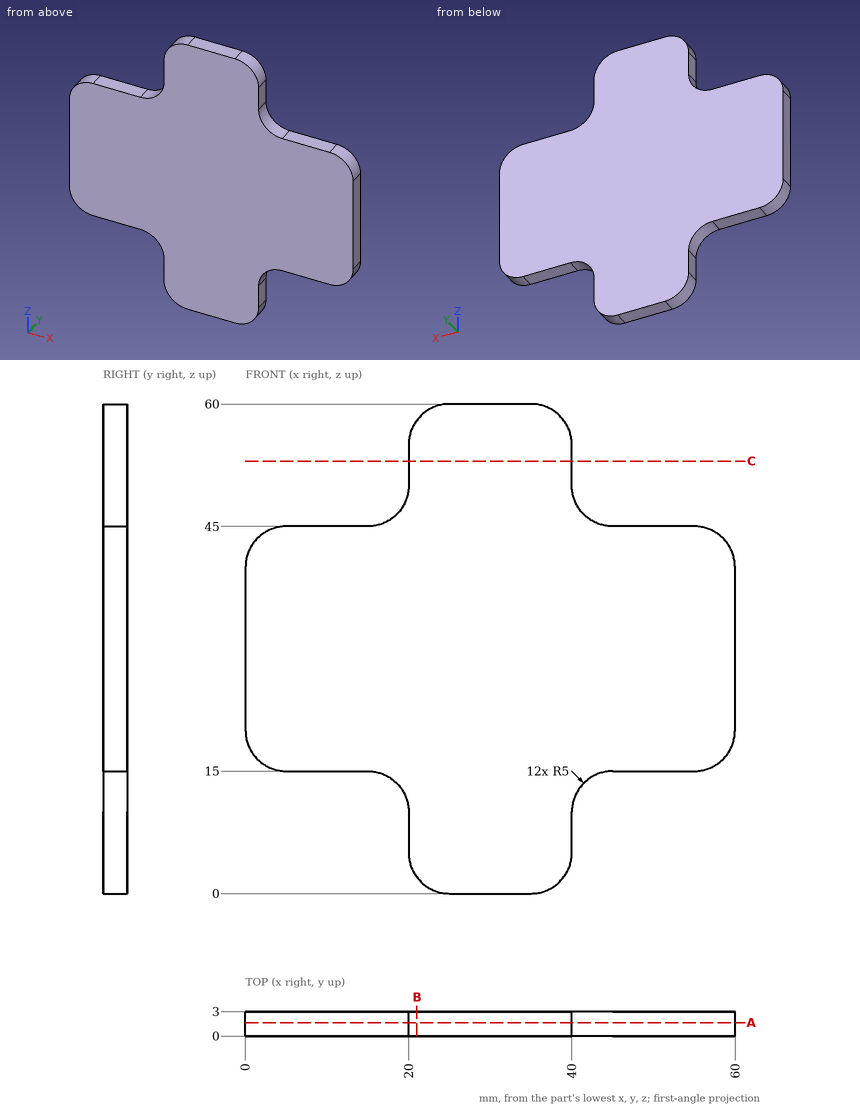
Geometry: see drawing. Coordinates: mm, zero at the bounding-box minimum. Give positions to 0.01 mm unless a question says otherwise; leave off trailing zeros. Order: outer loops, then holes, each group sorted by start corner. A loop starts at its lowest first (then second) coordinate and runs counter-clockwise, first axis right, second up. Notation, with made-up numbers: (3.25, 43) -> (37.25, 43) arc R13 cw to (37.25, 59) -> close; hole circle Ø10 at (38.5, 15.25). An arc over 180 degrees is marked (long way). Write each question's results on one line, items separated by ' | '.
1) Cut plane B-B (x = 21). Output: boundary loops of the cut face in (y, z), and give its area (3 significant figures).
Geometry says:
outline: (0, 2) -> (3, 2) -> (3, 58) -> (0, 58) -> close | area: 168 mm²
2) First-contact query: pin 1 Ø6 at (x, z) = (22, 53) entering from -Y; pin 2 Ø1.5 at (x, y) = (8.5, 1) entering from +Z. Flat tips, straight axial feed; report the tip coordinate or a pass-through.
Geometry says:
pin 1: stops at y = 0 | pin 2: stops at z = 45
3) Cut plane A-A (y = 1.65). Output: boundary loops of the cut face in (x, z), and give its area (3 significant figures).
Geometry says:
outline: (0, 20) arc R5 ccw to (5, 15) -> (15, 15) arc R5 cw to (20, 10) -> (20, 5) arc R5 ccw to (25, 0) -> (35, 0) arc R5 ccw to (40, 5) -> (40, 10) arc R5 cw to (45, 15) -> (55, 15) arc R5 ccw to (60, 20) -> (60, 40) arc R5 ccw to (55, 45) -> (45, 45) arc R5 cw to (40, 50) -> (40, 55) arc R5 ccw to (35, 60) -> (25, 60) arc R5 ccw to (20, 55) -> (20, 50) arc R5 cw to (15, 45) -> (5, 45) arc R5 ccw to (0, 40) -> close | area: 2,380 mm²
4) Line query: line 1 along X through (y, z) = (2.8, 6); line 2 along Z through (x, y) = (53.5, 0.55); line 3 along X through (y, z) = (1.2, 49). Output: solid intervals per line, ascending.
Geometry says:
line 1: x = 20 to 40 | line 2: z = 15 to 45 | line 3: x = 19.9 to 40.1
5) Cut plane C-C (z = 53). Output: boundary loops of the cut face in (x, y), and give its area (3 significant figures).
Geometry says:
outline: (20, 0) -> (40, 0) -> (40, 3) -> (20, 3) -> close | area: 60.0 mm²
